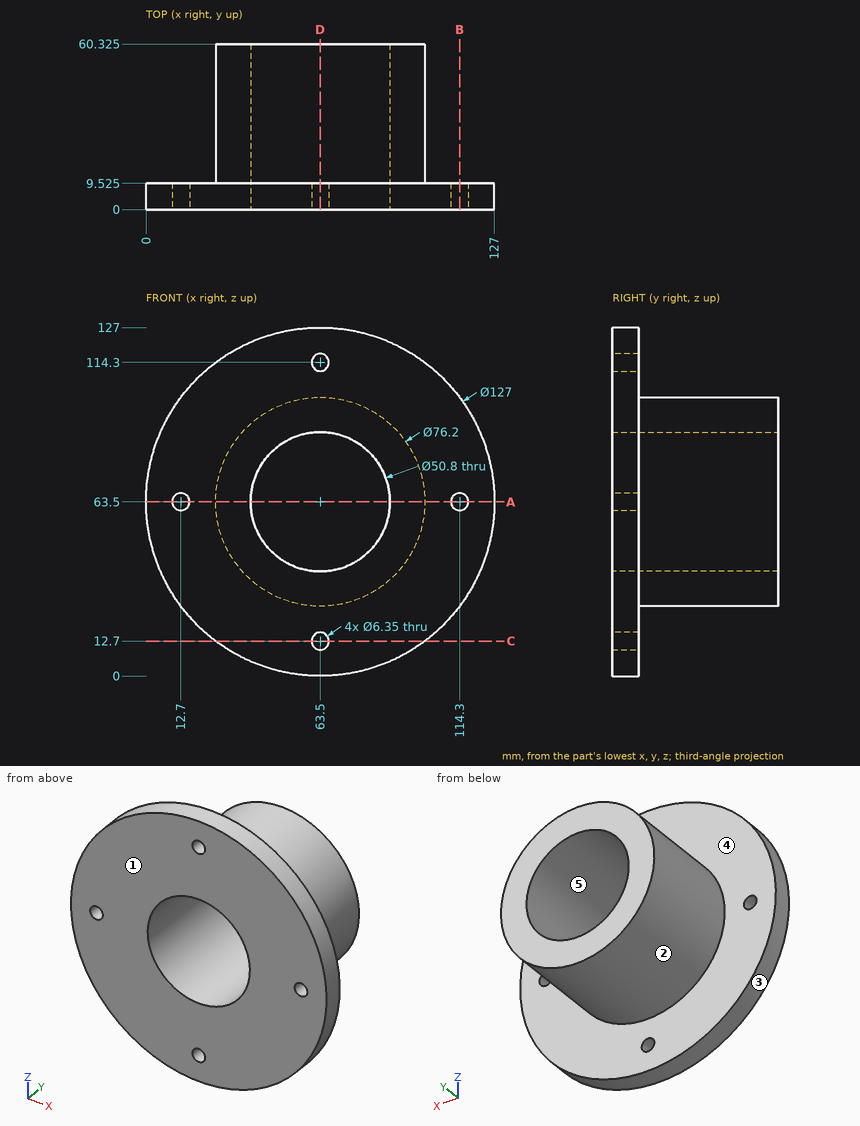
Here's the drawing with two shaded views (mm, measured from the low corner). I have some questions. A direction names the side the tool comes from. Give positions to 0.01 mm unless a question says otherwise; leave off trailing zeros. Loops run counter-clockwise (first coordinate to the right, second up) from the corner with the lowest first, then second, coordinate; pieces in that order, holes last. Notation, with made-up numbers: (53.5, 68.25) - (106.5, 68.25) arc R18 cw to (106.5, 96.25) - close; hole circle Ø2 at (-25.5, 24). An arc over 180 degrees is marked (long way). Answer in a Markdown table with one row per item. Add a question column.
Q1. For pin 1 (1.5 mm diameter, centred on x = 113, z = 83, fed in from +Y) (3 decimals); pin 2 (4 mm diameter, centred on x = 63.5, z = 114.3, fed in from +Y); pin 3 (5 mm diameter, centred on x = 93.5, y = 38, fed in from +Z); pin 4 (12 mm diameter, centred on y = 31, z = 49, fed in from +X), each with a flat end and sliding along its axis, tell me the tip position at first contact or that it passes through.
Q2. If we section it at B-B (x = 114.3): List the corners of the cut face in (y, z) for me (3 decimals).
Q3. If we section it at C-C (z = 12.7): List the corners of the cut face in (x, y) for me (3 decimals), plus the area to 3 significant figures.
Q4. If we section it at D-D (x = 63.5): List the corners of the cut face in (y, z) for me (3 decimals), plus the area to 3 significant figures.
Q5. We'd pull the mould along Z, two halves only. Please class the marked faces 3, 4 and 5: +Z half, -Z half, draft (parallel to the pull), parting line (faces both ways), or undercut.
Q6. Please list where these lines run through material, in increasing order: L1, parallel to X at y = 6, z = 63.5 (3 decimals); L2, parallel to X at y = 39.5, z = 63.5. Write a range as from..to.
Q7. Which directions (+Z, -Z, +X, -X, +Y, -Y) give clear straight access to the entire face, cutting with the end or side of a thin tool? Please do the marked faces 1 and 2.
Q8. If we section it at A-A (z = 63.5): List the corners of the cut face in (x, y) for me (3 decimals), plus the area to 3 significant figures.
The answers:
| question | item | result |
|---|---|---|
| 1 | pin 1 | stops at y = 9.525 |
| 1 | pin 2 | passes through |
| 1 | pin 3 | stops at z = 89.87 |
| 1 | pin 4 | stops at x = 100.64 |
| 2 | outline | (0, 25.4) - (9.525, 25.4) - (9.525, 60.325) - (0, 60.325) - close; (0, 66.675) - (9.525, 66.675) - (9.525, 101.6) - (0, 101.6) - close |
| 3 | outline | (25.4, 0) - (60.325, 0) - (60.325, 9.525) - (25.4, 9.525) - close; (66.675, 0) - (101.6, 0) - (101.6, 9.525) - (66.675, 9.525) - close |
| 3 | area | 665 mm^2 |
| 4 | outline | (0, 0) - (9.525, 0) - (9.525, 9.525) - (0, 9.525) - close; (0, 15.875) - (9.525, 15.875) - (9.525, 25.4) - (60.325, 25.4) - (60.325, 38.1) - (0, 38.1) - close; (0, 88.9) - (60.325, 88.9) - (60.325, 101.6) - (9.525, 101.6) - (9.525, 111.125) - (0, 111.125) - close; (0, 117.475) - (9.525, 117.475) - (9.525, 127) - (0, 127) - close |
| 4 | area | 1,900 mm^2 |
| 5 | face 3 | parting line |
| 5 | face 4 | draft |
| 5 | face 5 | undercut |
| 6 | L1 | x = 0..9.525, 15.875..38.1, 88.9..111.125, 117.475..127 |
| 6 | L2 | x = 25.4..38.1, 88.9..101.6 |
| 7 | face 1 | +Z, -Z, +X, -X, -Y |
| 7 | face 2 | +Y |
| 8 | outline | (0, 0) - (9.525, 0) - (9.525, 9.525) - (0, 9.525) - close; (15.875, 0) - (38.1, 0) - (38.1, 60.325) - (25.4, 60.325) - (25.4, 9.525) - (15.875, 9.525) - close; (88.9, 0) - (111.125, 0) - (111.125, 9.525) - (101.6, 9.525) - (101.6, 60.325) - (88.9, 60.325) - close; (117.475, 0) - (127, 0) - (127, 9.525) - (117.475, 9.525) - close |
| 8 | area | 1,900 mm^2 |
